```python
from build123d import *

# Parameters (mm, degrees)
SKETCH1_R           = 4.15
BOSS_EXTRUDE1_DEPTH = 3.2
SKETCH1_3_R         = 2.575
CUT_EXTRUDE1_DEPTH  = 1.8


with BuildPart() as part:
    # Sketch1 → Boss-Extrude1 (new body)
    with BuildSketch(Plane.XY.offset(17.54359624)):
        Polygon((8.498833186, -40.5), (-18.501166814, -40.5), (-18.501166814, -56.5), (-2.501166814, -56.5), (-2.501166814, -59), (8.498833186, -59), align=None)
        with Locations((4.246216621, -52.5)):
            Circle(SKETCH1_R, mode=Mode.SUBTRACT)
    extrude(amount=BOSS_EXTRUDE1_DEPTH)

    # Sketch2 → Cut-Revolve1 (revolve, cut)
    with BuildSketch(Plane(origin=(4.246216621, -52.5, 15.44359624), x_dir=(1, 0, 0), z_dir=(0, 1, 0)), mode=Mode.PRIVATE) as cut_revolve1_sk:
        Polygon((-3.899999957, -1.91392917), (-3.899999957, -3), (-4.335, -3), (-4.335, -2.846789772), align=None)
    revolve(cut_revolve1_sk.sketch.rotate(Axis((4.246216621, -52.5, 18.34359624), (0, 0, -1)), 180), axis=Axis((4.246216621, -52.5, 18.34359624), (0, 0, -1)), mode=Mode.SUBTRACT)

    # Sketch1_3 → Cut-Extrude1 (cut)
    with BuildSketch(Plane.XY.offset(17.54359624)):
        with Locations((-14.476166814, -44.525)):
            Circle(SKETCH1_3_R)
        with Locations((-6.526166814, -44.525)):
            Circle(SKETCH1_3_R)
        with Locations((-6.526166814, -52.475)):
            Circle(SKETCH1_3_R)
        with Locations((-14.476166814, -52.475)):
            Circle(SKETCH1_3_R)
    extrude(amount=CUT_EXTRUDE1_DEPTH, mode=Mode.SUBTRACT)


solid = part.part
```
CAD build for the part. Positions are in the model's coordinates, mm. A direction names the side the tool comes from. Round coordinates to 2 decimals unless told otherwise and drop trailing zeros. Loops run counter-clockwise (first coordinate to the right, second up) from the corner with the lowest first, then second, coordinate; pieces in that order, holes last. Notation, with made-up numbers: M -5.75,35.25 L 31.25,35.25 A11 cw 31.25,55.25 Z; hole C 26,6 d2. An arc over 180 degrees is marked long. Use a Markdown table: item, result. Add a question column.
(1) Cut at C-C (x = -4.5). Give the cut face in (y, z).
(2) Cut at A-A (z = 20.4). Give the cut face in (x, y), and give its area (3 significant figures).
(3) Drill centre lines: line 1 (X direction, y = -52.5, z = 18.4); line 2 (X direction, y = -43.75, z = 18.95); line 3 (Y direction, x = -12.5, z = 19.5). Where is each one in solid material? Low to high.
(4) Flat gauge pins, fed straight in: pin 1 (1.5 mm diameter, centred on x = -7.5, y = -45.5, fed in from -Z); pin 2 (1.2 mm diameter, centred on y = -58, z = 18.5, fed in from -X); pin 3 (5 mm diameter, centred on x = 4.25, y = -52.5, fed in from +Z). Where does each tip first touch, or does it go through?
(5) Which spindle directions (+Z, -Z, +X, -X, +Y, -Y) get a long thin tool onto all of the face, cutting with end or side? Do faces 1 (the face through (-11, -56.5, 19)), 2 (the face through (8.499, -50, 19)), 3 (the face through (-7, -52, 19.344)). Say none if no direction does.
(6) Pull direction X, two halves, no side cores. Call faces 4 (the face through (3.706, -48.385, 19.577)), 5 (the face through (-2.501, -58, 19)), 6 (the face through (-5, -40.5, 19)): +X half, -X half, draft (parallel to the pull), parting line (faces both ways), or undercut.
(7) Cut at D-D (y = -42.75). Give the cut face in (x, z), and give its area (3 significant figures).
(8) Cut at B-B (z = 18.75). Give the cut face in (x, y) (3 decimals), and give its area (3 significant figures).
Geometry says:
| question | item | result |
|---|---|---|
| 1 | outline | M -56.5,17.54 L -54.06,17.54 L -54.06,19.34 L -50.89,19.34 L -50.89,17.54 L -46.11,17.54 L -46.11,19.34 L -42.94,19.34 L -42.94,17.54 L -40.5,17.54 L -40.5,20.74 L -56.5,20.74 Z |
| 2 | outline | M -18.5,-56.5 L -2.5,-56.5 L -2.5,-59 L 8.5,-59 L 8.5,-40.5 L -18.5,-40.5 Z; hole C 4.25,-52.5 d8.3 |
| 2 | area | 405 mm² |
| 3 | line 1 | x = -18.5 to -17.05, -11.9 to -9.1, -3.95 to -0.09 |
| 3 | line 2 | x = -18.5 to -16.93, -12.02 to -8.98, -4.07 to 8.5 |
| 3 | line 3 | y = -56.5 to -40.5 |
| 4 | pin 1 | stops at z = 19.34 |
| 4 | pin 2 | stops at x = -2.5 |
| 4 | pin 3 | passes through |
| 5 | face 1 | +Z, -Z, -X, -Y |
| 5 | face 2 | +Z, -Z, +X, +Y, -Y |
| 5 | face 3 | -Z |
| 6 | face 4 | undercut |
| 6 | face 5 | -X half |
| 6 | face 6 | draft |
| 7 | outline | M -18.5,17.54 L -16.34,17.54 L -16.34,19.34 L -12.61,19.34 L -12.61,17.54 L -8.39,17.54 L -8.39,19.34 L -4.66,19.34 L -4.66,17.54 L 8.5,17.54 L 8.5,20.74 L -18.5,20.74 Z |
| 7 | area | 73.0 mm² |
| 8 | outline | M -18.501,-56.5 L -2.501,-56.5 L -2.501,-59 L 8.499,-59 L 8.499,-40.5 L -18.501,-40.5 Z; hole C -14.476,-52.475 d5.15; hole C -14.476,-44.525 d5.15; hole C -6.526,-52.475 d5.15; hole C -6.526,-44.525 d5.15; hole C 4.246,-52.5 d8.3 |
| 8 | area | 322 mm² |
